Autodesk Inventor part; units mm, degrees
ref_plane "YZ Plane" through (0, 0, 0) normal (1, 0, 0) x (0, 1, 0)
ref_plane "XZ Plane" through (0, 0, 0) normal (0, 1, 0) x (-1, 0, 0)
ref_plane "XY Plane" through (0, 0, 0) normal (0, 0, 1) x (1, 0, 0)
ref_plane "Work Plane1" through (0, 0, 0) normal (0, 0, 1) x (1, 0, 0)
sketch "Sketch2" plane through (0, 0, 0) normal (0, 0, 1) x (1, 0, 0)
  line L0 (22.5, 31) -> (-17.5, 31)
  line L1 (-17.5, 31) -> (-17.5, 16)
  line L2 (-17.5, 16) -> (22.5, 16)
  line L3 (22.5, 16) -> (22.5, 31)
  point P0 (0, 0)
  dimension "d1" = 15
  dimension "d4" = 40
  dimension "d5" = 22.5
  dimension "d6" = 31
extrude "Extrusion1" add sketch "Sketch2" along normal blind 2
hole "Hole1" at (-14.5, 23.5, 0) direction (0, 0, 1) diameter 3 end through all
hole "Hole2" at (-1.5, 23.5, 0) direction (0, 0, 1) diameter 3 end through all
equation "\"d8\" = 0.5 * d1"
equation "\"d17\" = 0.5 * d1"
properties part number "HTD-5M-belt-clamp" material "Aluminum 6061"
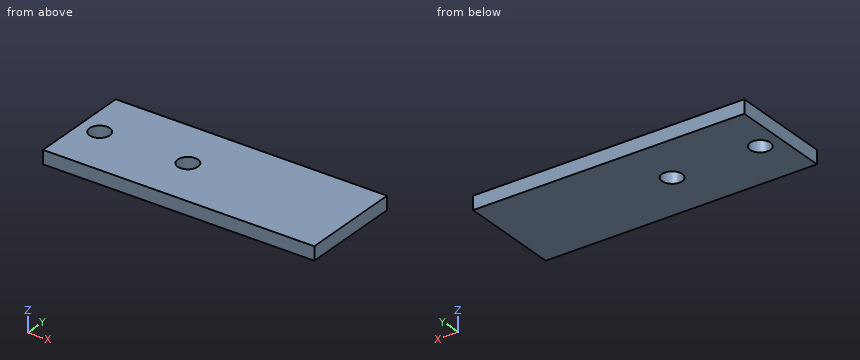
Work out the finished part from the listing and answer in its coordinate system (mm). Give positions to 0.01 mm unless a question says otherwise; leave off trailing zeros. Loops run counter-clockwise (first coordinate to the right, second up) from the corner with the lowest first, then second, coordinate; pieces in that order, holes last. Notation, with made-up numbers: (-1.75, 38.25) -> (18.25, 38.25) arc R23 ccw to (18.25, 57.25) -> close; hole circle Ø6 at (58.5, 72). An arc over 180 degrees is marked (long way). Use a Markdown table: item, result. Add a question column.
1) Consider line 1 along X through (y, z) = (23.5, 1); line 2 along X through (y, z) = (24, 0.75); line 3 along Y through (x, z) = (-2, 0.2). Determine where each line is inside the solid, lowest interval first.
2) The part is cut by section C-C, the plane z = 1.5. Determine the outline of the cut face in (x, y), plus the area to 3 significant figures.
3) Each of these flat-tipped pins is pushed along its axis until it touches: P1, Ø2.5, axis at x = -1.5, y = 23.5, coming from the -Z side; P2, Ø6, axis at x = 11, y = 29, coming from the -Z side. Where does it stop, or does it pass through?
4) The part is cut by section A-A, the plane y = 23.5. Determine the outline of the cut face in (x, z), plus the area to 3 significant figures.
5) The part is cut by section B-B, the plane x = -14.5. Determine the outline of the cut face in (y, z).
6) The part is cut by section D-D, the plane x = -0.5. Determine the outline of the cut face in (y, z).
Reported:
| question | item | result |
|---|---|---|
| 1 | line 1 | x = -17.5 to -16, -13 to -3, 0 to 22.5 |
| 1 | line 2 | x = -17.5 to -15.91, -13.09 to -2.91, -0.09 to 22.5 |
| 1 | line 3 | y = 16 to 22.09, 24.91 to 31 |
| 2 | outline | (-17.5, 16) -> (22.5, 16) -> (22.5, 31) -> (-17.5, 31) -> close; hole circle Ø3 at (-14.5, 23.5); hole circle Ø3 at (-1.5, 23.5) |
| 2 | area | 586 mm^2 |
| 3 | P1 | passes through |
| 3 | P2 | stops at z = 0 |
| 4 | outline | (-17.5, 0) -> (-16, 0) -> (-16, 2) -> (-17.5, 2) -> close; (-13, 0) -> (-3, 0) -> (-3, 2) -> (-13, 2) -> close; (0, 0) -> (22.5, 0) -> (22.5, 2) -> (0, 2) -> close |
| 4 | area | 68.0 mm^2 |
| 5 | outline | (16, 0) -> (22, 0) -> (22, 2) -> (16, 2) -> close; (25, 0) -> (31, 0) -> (31, 2) -> (25, 2) -> close |
| 6 | outline | (16, 0) -> (22.38, 0) -> (22.38, 2) -> (16, 2) -> close; (24.62, 0) -> (31, 0) -> (31, 2) -> (24.62, 2) -> close |
